Build history of the part. All positions in model axes, mm. A direction names the side the tool comes from. Round coordinates to 2 decimals unless told otherwise and drop trailing zeros. Loops run counter-clockwise (first coordinate to the right, second up) from the corner with the lowest first, then second, coordinate; pieces in that order, holes last.
from build123d import *

# Parameters (mm, degrees)
BOSS_EXTRUDE1_DEPTH = 10
SKETCH2_R           = 4
CUT_EXTRUDE1_DEPTH  = 5


with BuildPart() as part:
    # Sketch1 → Boss-Extrude1 (new body)
    with BuildSketch(Plane(origin=(0, 0, 0), x_dir=(1, 0, 0), z_dir=(0, 1, 0))):
        Polygon((2.781569966, 65), (2.781569966, 5), (7.781569966, 0), (67.781569966, 0), (72.781569966, 5), (72.781569966, 65), (67.781569966, 70), (7.781569966, 70), align=None)
        with BuildLine():
            ThreePointArc((12.781569966, 57), (10.660249622, 62.121320344), (15.781569966, 60))
            Line((15.781569966, 60), (59.781569966, 60))
            ThreePointArc((59.781569966, 60), (62.781569966, 63), (65.781569966, 60))
            ThreePointArc((65.781569966, 60), (64.902890309, 57.878679656), (62.781569966, 57))
            Line((62.781569966, 57), (62.781569966, 13))
            ThreePointArc((62.781569966, 13), (64.902890309, 12.121320344), (65.781569966, 10))
            ThreePointArc((65.781569966, 10), (62.781569966, 7), (59.781569966, 10))
            Line((59.781569966, 10), (15.781569966, 10))
            ThreePointArc((15.781569966, 10), (10.660249622, 7.878679656), (12.781569966, 13))
            Line((12.781569966, 13), (12.781569966, 57))
        make_face(mode=Mode.SUBTRACT)
    extrude(amount=BOSS_EXTRUDE1_DEPTH)

    # Sketch2 → Cut-Extrude1 (cut)
    with BuildSketch(Plane.XZ):
        with Locations((22.781569966, -5)):
            Circle(SKETCH2_R)
        with Locations((52.681064902, -5)):
            Circle(SKETCH2_R)
        with Locations((67.781569966, -20)):
            Circle(SKETCH2_R)
        with Locations((67.781569966, -50)):
            Circle(SKETCH2_R)
        with Locations((52.681064902, -64.899494937)):
            Circle(SKETCH2_R)
        with Locations((22.781569966, -64.899494937)):
            Circle(SKETCH2_R)
        with Locations((7.831822498, -50)):
            Circle(SKETCH2_R)
        with Locations((7.831822498, -20)):
            Circle(SKETCH2_R)
    extrude(amount=-CUT_EXTRUDE1_DEPTH, mode=Mode.SUBTRACT)


solid = part.part
(1) Slice it at C-C on y = 4. Count the separate pieces of the cut face and the enclosed holes in it, plus the area to 3 significant figures.
Responses:
separate pieces: 1
enclosed holes: 9
area: 1,860 mm2
(2) Slice it at A-A on z = -37. List the corners of the cut face in (x, y).
Responses:
outline: (2.78, 0) - (12.78, 0) - (12.78, 10) - (2.78, 10) - close; (62.78, 0) - (72.78, 0) - (72.78, 10) - (62.78, 10) - close
(3) Which spindle directions (+Z, -Z, +X, -X, +Y, -Y) get a long thin tool onto all of the face, cutting with end or side? Do faces 1 (the face through (71.597, 2.465, -18.799)), 2 (the face through (72.782, 5, -35)). Say none if no direction does.
Responses:
face 1: -Y
face 2: +Z, -Z, +X, +Y, -Y
(4) Pin check, flat tip, straight feed: P1, Ø4, axis at x = 21, z = -5, coming from the -Y side. Stop position of the tip, or through.
Responses:
P1: stops at y = 5
(5) Slice it at D-D on z = -20. List the corners of the cut face in (x, y).
Responses:
outline: (2.78, 0) - (3.83, 0) - (3.83, 5) - (11.83, 5) - (11.83, 0) - (12.78, 0) - (12.78, 10) - (2.78, 10) - close; (62.78, 0) - (63.78, 0) - (63.78, 5) - (71.78, 5) - (71.78, 0) - (72.78, 0) - (72.78, 10) - (62.78, 10) - close
(6) Probe line 1 (X direction, y = 6, z = -19); line 2 (Z direction, x = 34, y = 8); line 3 (X direction, y = 4, z = -19). List the from-to ranges inside material, lowest first.
Responses:
line 1: x = 2.78 to 12.78, 62.78 to 72.78
line 2: z = -70 to -60, -10 to 0
line 3: x = 2.78 to 3.96, 11.7 to 12.78, 62.78 to 63.91, 71.65 to 72.78
(7) Pull direction Z, two halves, no side cores. Call faces 3 (the face through (12.782, 5, -35)), 4 (the face through (38, 0, -9)), 5 (the face through (70.25, 4.93, -2.47)): +Z half, -Z half, draft (parallel to the pull), parting line (faces both ways), or undercut.
Responses:
face 3: undercut
face 4: draft
face 5: +Z half
(8) Slice it at B-B on y = 7.75. List the corners of the cut face in (x, z), plus the area to 3 significant figures.
Responses:
outline: (2.78, -65) - (7.78, -70) - (67.78, -70) - (72.78, -65) - (72.78, -5) - (67.78, 0) - (7.78, 0) - (2.78, -5) - close; hole (12.78, -57) arc R3 ccw (long way) to (15.78, -60) - (59.78, -60) arc R3 ccw (long way) to (62.78, -57) - (62.78, -13) arc R3 ccw (long way) to (59.78, -10) - (15.78, -10) arc R3 ccw (long way) to (12.78, -13) - close
area: 2,270 mm2
